Can you work these out from the drawing? Everything is in mm from the part's minimum corner. A direction names the side the tool comes from. Coordinates: 2 decimals unless noted, no trailing zeros. Write each loop counter-clockwise with the first axis right and the second up, starting at its lowest first coordinate (ties: lowest second). Pieces come first, ordered by that corner, then holes.
(1) Imagine slicing it at C-C, the plane x = 3. List the corners of the cut face in (y, z) for me (1 decimal), plus the area to 3 significant figures.
(2) Which directions (+Z, -Z, +X, -X, +Y, -Y) give clear straight access to the entire face, cutting with the end or side of a thin tool? Please do the marked faces 1, 2 and 3.
(3) Imagine slicing it at A-A, the plane x = 15.5. List the corners of the cut face in (y, z) for me (1 decimal).
(4) Imagine slicing it at B-B, the plane z = 17. List the corners of the cut face in (x, y) for me (1 decimal), plus the area to 3 significant figures.
(5) Thinking about a two-plate mould opening in X: for the marked faces 4, 5, 6 and 7, which applies, released by +X, released by -X, zero draft, split by the parting line, or undercut?
(6) Please list where these lines run through material, in increasing order: probe 1 along Y at (x, z) = (27.5, 5.5); probe 2 along X at (y, z) = (8.75, 18) (1 decimal); probe 3 along Z at (x, y) = (5, 12).
(7) For pin 1 Ø1.5 at (x, y) = (4.5, 9) entering from -Z; pin 2 Ø6 at (x, y) = (25.5, 13) entering from +Z; pin 3 Ø6.5 at (x, z) = (13, 5) entering from +Y, each with a flat end and sliding along its axis, tell me the tip position at first contact or that it passes through.
(8) Imagine slicing it at D-D, the plane y = 4.25. List the corners of the cut face in (x, z) for me (1 decimal), plus the area to 3 significant figures.
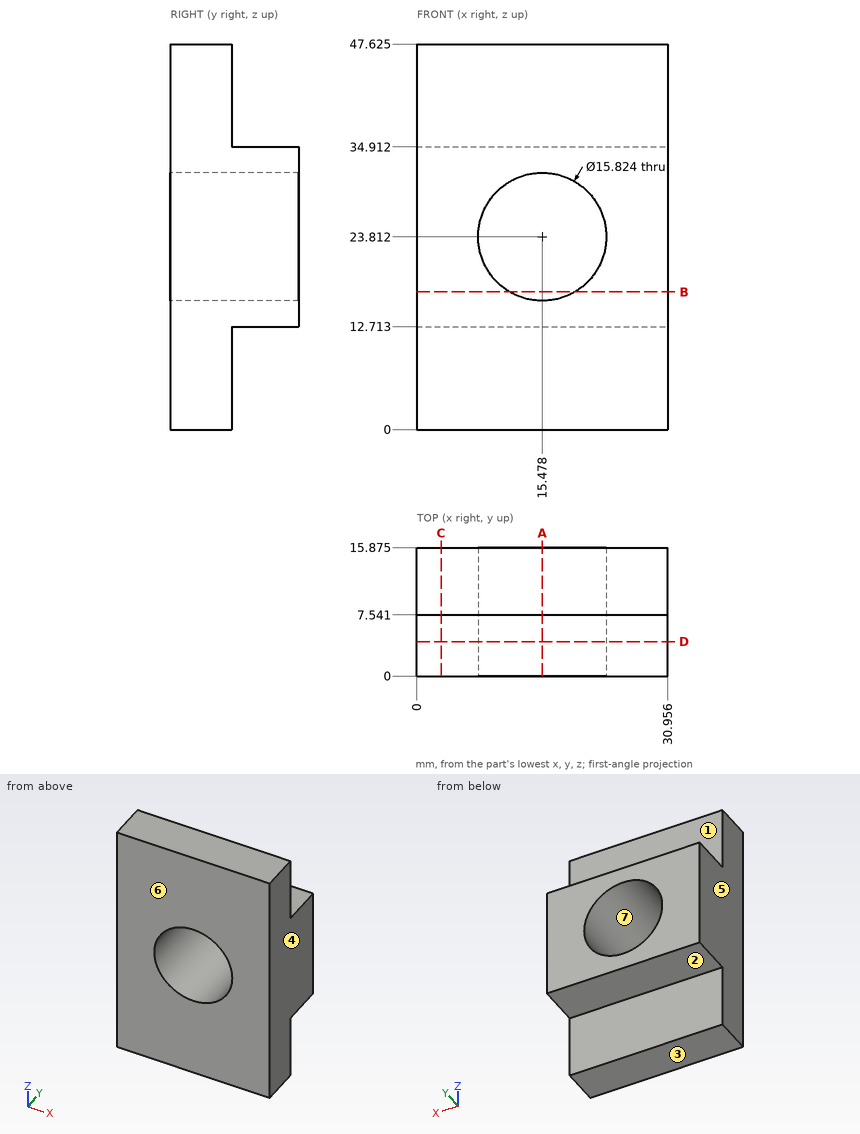
Recorded:
1. outline: (0, 0) - (7.5, 0) - (7.5, 12.7) - (15.9, 12.7) - (15.9, 34.9) - (7.5, 34.9) - (7.5, 47.6) - (0, 47.6) - close
1. area: 544 mm2
2. face 1: +Z, +X, -X, +Y
2. face 2: -Z, +X, -X, +Y
2. face 3: -Z, +X, -X, +Y, -Y
3. outline: (0, 0) - (7.5, 0) - (7.5, 12.7) - (15.9, 12.7) - (15.9, 15.9) - (0, 15.9) - close; (0, 31.7) - (15.9, 31.7) - (15.9, 34.9) - (7.5, 34.9) - (7.5, 47.6) - (0, 47.6) - close
4. outline: (0, 0) - (11.5, 0) - (11.5, 15.9) - (0, 15.9) - close; (19.5, 0) - (31, 0) - (31, 15.9) - (19.5, 15.9) - close
4. area: 364 mm2
5. face 4: released by +X
5. face 5: released by -X
5. face 6: zero draft
5. face 7: undercut
6. probe 1: y = 0 to 7.54
6. probe 2: x = 0 to 10.1, 20.8 to 31
6. probe 3: z = 12.71 to 34.91
7. pin 1: stops at z = 12.71
7. pin 2: stops at z = 34.91
7. pin 3: stops at y = 7.54
8. outline: (0, 0) - (31, 0) - (31, 47.6) - (0, 47.6) - close; hole circle Ø15.8 at (15.5, 23.8)
8. area: 1,280 mm2
